The listing builds one solid part. Answer for the finished solid, in the listing's coordinates (mm). Face numbers are marked on the shaded views. A direction names the side the tool comes from. Round coordinates to 2 decimals unless told otherwise and drop trailing zeros.
Item 1: Find section C-C on x = 14. Give the number of separate pieces and of enclosed holes in the cut face, then the cut area to 3 significant figures.
Item 2: A tool of negligible diameter and unlimited length cuts with its end or side. For the marked faces 1, 2 and 3, from which of +Z, -Z, +X, -X, +Y, -Y can it reach the whole face along a straight path? Write none if from no direction.
Item 3: Find the intervals of material crossed by probe 1 along Z at (x, y) = (15, 68.5); probe 2 along Y at (x, z) = (16.5, 0) (3 decimals); probe 3 along X at (y, z) = (69, -17), in increasing order.
Item 4: Each of these flat-tipped pins is pushed along its axis until it touches: pin 1 (1.5 mm diameter, centred on y = 69, z = -12.5, fed in from -X); pin 2 (1 mm diameter, centred on y = 66, z = -2, fed in from -X); pin 3 (7 mm diameter, centred on x = 14.93, z = -16.83, fed in from -Y) (3 decimals); pin 4 (5 mm diameter, centred on x = 5.5, z = 14.5, fed in from -Y). Where does it stop, or does it pass through?
Item 5: For a pull along X with two mould halves and no side action, classify the marked faces 4 and 5 as +X half, -X half, draft (parallel to the pull), parting line (faces both ways), or undercut.
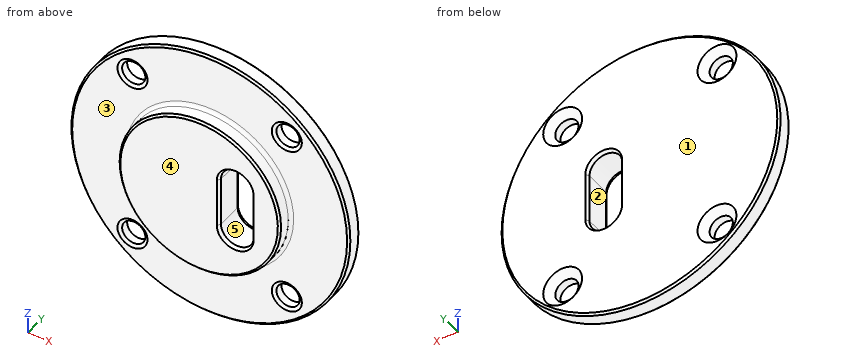
```python
from build123d import *
from OCP.BRepFilletAPI import BRepFilletAPI_MakeChamfer

# Parameters (mm, degrees)
STOCK_DGT_START                               = 66.675
STOCK_DGT_INSIDE_SWERVE_STRUCTURE_SM_2_R      = 26.9875
STOCK_DGT_INSIDE_SWERVE_STRUCTURE_SM_2_R_2    = 2.2479
STOCK_DGT_INSIDE_SWERVE_STRUCTURE_SMALL_DEPTH = 3.175
STOCK_DGT_START_2                             = 63.5
STOCK_DGT_INSIDE_SWERVE_STRUCTURE_SM_3_O_R    = 15.875
STOCK_DGT_INSIDE_SWERVE_STRUCTURE_SM_3_DEPTH  = 3.175
SKETCH1_R                                     = 15.875
SKETCH1_R_2                                   = 15.621
CUT_EXTRUDE1_DEPTH                            = 3.175
FILLET1_R                                     = 0.635
CHAMFER1_SIZE                                 = 0.381
CHAMFER2_SIZE                                 = 0.381
CHAMFER2_SIZE2                                = 0.659911358
CHAMFER3_SIZE                                 = 1.27
CHAMFER3_SIZE2                                = 1.513527063


# Read off the part's stored shape, not the designer's step: Stock-DGT inside swerve structure Small Bearing-1
with BuildPart() as part:
    # Stock-DGT inside swerve structure Sm 2 → Stock-DGT inside swerve structure Small Bearing-1 (new body)
    with BuildSketch(Plane(origin=(0, 0, 0), x_dir=(1, 0, 0), z_dir=(0, 1, 0)).offset(STOCK_DGT_START)):
        Circle(STOCK_DGT_INSIDE_SWERVE_STRUCTURE_SM_2_R)
        with Locations((-14.933176064, -16.8275)):
            Circle(STOCK_DGT_INSIDE_SWERVE_STRUCTURE_SM_2_R_2, mode=Mode.SUBTRACT)
        with Locations((14.933176064, -16.8275)):
            Circle(STOCK_DGT_INSIDE_SWERVE_STRUCTURE_SM_2_R_2, mode=Mode.SUBTRACT)
        with Locations((-14.933176064, 16.8275)):
            Circle(STOCK_DGT_INSIDE_SWERVE_STRUCTURE_SM_2_R_2, mode=Mode.SUBTRACT)
        with Locations((14.933176064, 16.8275)):
            Circle(STOCK_DGT_INSIDE_SWERVE_STRUCTURE_SM_2_R_2, mode=Mode.SUBTRACT)
        with BuildLine():
            Line((3.81, -4.7625), (3.81, 4.7625))
            ThreePointArc((3.81, 4.7625), (6.985, 7.9375), (10.16, 4.7625))
            Line((10.16, 4.7625), (10.16, -4.7625))
            ThreePointArc((10.16, -4.7625), (6.985, -7.9375), (3.81, -4.7625))
        make_face(mode=Mode.SUBTRACT)
    extrude(amount=STOCK_DGT_INSIDE_SWERVE_STRUCTURE_SMALL_DEPTH)

    # Stock-DGT inside swerve structure Sm 3 o → Stock-DGT inside swerve structure Sm 3 (add)
    with BuildSketch(Plane(origin=(0, 0, 0), x_dir=(1, 0, 0), z_dir=(0, 1, 0)).offset(STOCK_DGT_START_2)):
        Circle(STOCK_DGT_INSIDE_SWERVE_STRUCTURE_SM_3_O_R)
        with BuildLine():
            ThreePointArc((10.16, -4.7625), (6.985, -7.9375), (3.81, -4.7625))
            Line((3.81, -4.7625), (3.81, 4.7625))
            ThreePointArc((3.81, 4.7625), (6.985, 7.9375), (10.16, 4.7625))
            Line((10.16, 4.7625), (10.16, -4.7625))
        make_face(mode=Mode.SUBTRACT)
    extrude(amount=STOCK_DGT_INSIDE_SWERVE_STRUCTURE_SM_3_DEPTH)

    # Sketch1 → Cut-Extrude1 (cut)
    with BuildSketch(Plane.XZ.offset(-63.5)):
        Circle(SKETCH1_R)
        with Locations(Location((0, 0, 0), (0, 0, 270))):
            Circle(SKETCH1_R_2, mode=Mode.SUBTRACT)
    extrude(amount=-CUT_EXTRUDE1_DEPTH, mode=Mode.SUBTRACT)

    # Fillet1
    fillet1_edges = [part.edges().sort_by_distance(p)[0] for p in [
        (0, 66.675, 15.621),
    ]]
    fillet(fillet1_edges, radius=FILLET1_R)

    # Chamfer1
    chamfer1_edges = [part.edges().sort_by_distance(p)[0] for p in [
        (-26.9875, 66.675, 0),
        (-26.9875, 69.85, 0),
        (0, 63.5, 15.621),
    ]]
    chamfer(chamfer1_edges, length=CHAMFER1_SIZE)

    # Chamfer2: one chamfer whose edges measure the first distance from different faces: ONE call of the kernel's chamfer builder (chamfer() names one face for all edges)
    chamfer2_edges_1 = [part.edges().sort_by_distance(p)[0] for p in [
        (-17.181076064, 66.675, -16.8275),
    ]]
    chamfer2_side_1 = [part.faces().sort_by_distance(p)[0] for p in [
        (-17.181076064, 68.2625, -16.8275),
    ]]
    chamfer2_edges_2 = [part.edges().sort_by_distance(p)[0] for p in [
        (-17.181076064, 66.675, 16.8275),
    ]]
    chamfer2_side_2 = [part.faces().sort_by_distance(p)[0] for p in [
        (-17.181076064, 68.2625, 16.8275),
    ]]
    chamfer2_edges_3 = [part.edges().sort_by_distance(p)[0] for p in [
        (10.16, 63.5, 0),
        (6.985, 63.5, -7.9375),
        (3.81, 63.5, 0),
        (6.985, 63.5, 7.9375),
    ]]
    chamfer2_side_3 = [part.faces().sort_by_distance(p)[0] for p in [
        (-1.009698226, 63.5, 0),
    ]]
    chamfer2_edges_4 = [part.edges().sort_by_distance(p)[0] for p in [
        (6.985, 69.85, 7.9375),
        (10.16, 69.85, 0),
        (6.985, 69.85, -7.9375),
        (3.81, 69.85, 0),
    ]]
    chamfer2_side_4 = [part.faces().sort_by_distance(p)[0] for p in [
        (-0.311216165, 69.85, 0),
    ]]
    chamfer2_edges_5 = [part.edges().sort_by_distance(p)[0] for p in [
        (12.685276064, 66.675, 16.8275),
    ]]
    chamfer2_side_5 = [part.faces().sort_by_distance(p)[0] for p in [
        (12.685276064, 68.2625, 16.8275),
    ]]
    chamfer2_edges_6 = [part.edges().sort_by_distance(p)[0] for p in [
        (12.685276064, 66.675, -16.8275),
    ]]
    chamfer2_side_6 = [part.faces().sort_by_distance(p)[0] for p in [
        (12.685276064, 68.2625, -16.8275),
    ]]
    chamfer2 = BRepFilletAPI_MakeChamfer(part.part.solid().wrapped)
    for e in chamfer2_edges_1:
        chamfer2.Add(CHAMFER2_SIZE, CHAMFER2_SIZE2, e.wrapped, chamfer2_side_1[0].wrapped)  # the first distance lies on this face
    for e in chamfer2_edges_2:
        chamfer2.Add(CHAMFER2_SIZE, CHAMFER2_SIZE2, e.wrapped, chamfer2_side_2[0].wrapped)  # the first distance lies on this face
    for e in chamfer2_edges_3:
        chamfer2.Add(CHAMFER2_SIZE, CHAMFER2_SIZE2, e.wrapped, chamfer2_side_3[0].wrapped)  # the first distance lies on this face
    for e in chamfer2_edges_4:
        chamfer2.Add(CHAMFER2_SIZE, CHAMFER2_SIZE2, e.wrapped, chamfer2_side_4[0].wrapped)  # the first distance lies on this face
    for e in chamfer2_edges_5:
        chamfer2.Add(CHAMFER2_SIZE, CHAMFER2_SIZE2, e.wrapped, chamfer2_side_5[0].wrapped)  # the first distance lies on this face
    for e in chamfer2_edges_6:
        chamfer2.Add(CHAMFER2_SIZE, CHAMFER2_SIZE2, e.wrapped, chamfer2_side_6[0].wrapped)  # the first distance lies on this face
    add(Compound.cast(chamfer2.Shape()), mode=Mode.REPLACE)

    # Chamfer3: one chamfer whose edges measure the first distance from different faces: ONE call of the kernel's chamfer builder (chamfer() names one face for all edges)
    chamfer3_edges_1 = [part.edges().sort_by_distance(p)[0] for p in [
        (-17.181076064, 69.85, -16.8275),
    ]]
    chamfer3_side_1 = [part.faces().sort_by_distance(p)[0] for p in [
        (-17.181076064, 68.453, -16.8275),
    ]]
    chamfer3_edges_2 = [part.edges().sort_by_distance(p)[0] for p in [
        (-17.181076064, 69.85, 16.8275),
    ]]
    chamfer3_side_2 = [part.faces().sort_by_distance(p)[0] for p in [
        (-17.181076064, 68.453, 16.8275),
    ]]
    chamfer3_edges_3 = [part.edges().sort_by_distance(p)[0] for p in [
        (12.685276064, 69.85, 16.8275),
    ]]
    chamfer3_side_3 = [part.faces().sort_by_distance(p)[0] for p in [
        (12.685276064, 68.453, 16.8275),
    ]]
    chamfer3_edges_4 = [part.edges().sort_by_distance(p)[0] for p in [
        (12.685276064, 69.85, -16.8275),
    ]]
    chamfer3_side_4 = [part.faces().sort_by_distance(p)[0] for p in [
        (12.685276064, 68.453, -16.8275),
    ]]
    chamfer3 = BRepFilletAPI_MakeChamfer(part.part.solid().wrapped)
    for e in chamfer3_edges_1:
        chamfer3.Add(CHAMFER3_SIZE, CHAMFER3_SIZE2, e.wrapped, chamfer3_side_1[0].wrapped)  # the first distance lies on this face
    for e in chamfer3_edges_2:
        chamfer3.Add(CHAMFER3_SIZE, CHAMFER3_SIZE2, e.wrapped, chamfer3_side_2[0].wrapped)  # the first distance lies on this face
    for e in chamfer3_edges_3:
        chamfer3.Add(CHAMFER3_SIZE, CHAMFER3_SIZE2, e.wrapped, chamfer3_side_3[0].wrapped)  # the first distance lies on this face
    for e in chamfer3_edges_4:
        chamfer3.Add(CHAMFER3_SIZE, CHAMFER3_SIZE2, e.wrapped, chamfer3_side_4[0].wrapped)  # the first distance lies on this face
    add(Compound.cast(chamfer3.Shape()), mode=Mode.REPLACE)


solid = part.part
```
Check values:
1. separate pieces: 3
1. enclosed holes: 0
1. area: 160 mm2
2. face 1: +Z, -Z, +X, -X, +Y
2. face 2: +Y, -Y
2. face 3: -Y
3. probe 1: z = -22.43 to -19.07, -14.58 to 14.58, 19.07 to 22.43
3. probe 2: y = 66.675 to 69.85
3. probe 3: x = -20.96 to -17.68, -12.19 to 12.19, 17.68 to 20.96
4. pin 1: stops at x = -24.3
4. pin 2: stops at x = -15.7
4. pin 3: stops at y = 66.675
4. pin 4: stops at y = 63.5
5. face 4: draft
5. face 5: undercut
